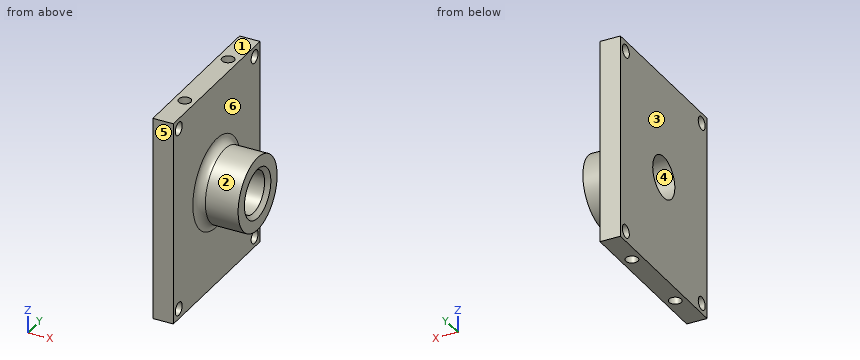
Autodesk Inventor part; units mm, degrees
ref_plane "YZ Plane" through (0, 0, 0) normal (1, 0, 0) x (0, 1, 0)
ref_plane "XZ Plane" through (0, 0, 0) normal (0, 1, 0) x (-1, 0, 0)
ref_plane "XY Plane" through (0, 0, 0) normal (0, 0, 1) x (1, 0, 0)
sketch "Sketch1" plane through (0, 0, 0) normal (1, 0, 0) x (0, 1, 0)
  line L0 (20, 25) -> (-20, 25)
  line L1 (-20, 25) -> (-20, -25)
  line L2 (-20, -25) -> (20, -25)
  line L3 (20, -25) -> (20, 25)
  point P0 (0, 0)
  dimension "d0" = 40
  dimension "d1" = 50
  dimension "d2" = 20
  dimension "d3" = 25
extrude "Extrusion1" add sketch "Sketch1" along normal blind 5
sketch "Sketch2" plane through (5, 0, 0) normal (1, 0, 0) x (0, 0, -1)
  circle A0 centre (0, 0) radius 5.1
  dimension "d6" = 10.2
extrude "Extrusion2" cut sketch "Sketch2" against normal through all
sketch "Sketch3" plane through (5, 0, 0) normal (1, 0, 0) x (0, 0, -1)
  circle A0 centre (0, 0) radius 5.1
  circle A1 centre (0, 0) radius 9
  dimension "d9" = 10.2
  dimension "d10" = 18
extrude "Extrusion3" add sketch "Sketch3" along normal blind 10
chamfer "Chamfer1" distance 1 angle 45 1 edges at (15, 0, 5.1)
fillet "Fillet1" radius 2 1 edges at (5, 0, 9)
sketch "Sketch4" plane through (5, 0, 0) normal (1, 0, 0) x (0, 0, -1)
  circle A0 centre (-22.5, 17.5) radius 1.6
  circle A1 centre (22.5, 17.5) radius 1.6
  circle A2 centre (22.5, -17.5) radius 1.6
  circle A3 centre (-22.5, -17.5) radius 1.6
  line L0 (-25, 20) -> (-25, -20)
  line L1 (25, 20) -> (-25, 20)
  line L2 (25, -20) -> (25, 20)
  line L3 (-25, -20) -> (25, -20)
  point P0 (0, 0)
  dimension "d17" = 3.2
  dimension "d18" = 3.2
  dimension "d19" = 3.2
  dimension "d20" = 3.2
  dimension "d21" = 2.5
  dimension "d22" = 2.5
  dimension "d23" = 2.5
  dimension "d24" = 2.5
  dimension "d25" = 2.5
  dimension "d26" = 2.5
  dimension "d27" = 2.5
  dimension "d28" = 2.5
extrude "Extrusion4" cut sketch "Sketch4" against normal through all contours A0 | A1 | A2 | A3
sketch "Sketch5" plane through (0, -20, 25) normal (0, 0, 1) x (1, 0, 0)
  circle A0 centre (2.5, 30) radius 1.5
  line L0 (0, 40) -> (0, 0)
  circle A1 centre (2.5, 10) radius 1.5
  point P0 (0, 20)
  point P1 (0, 20)
  point P2 (0, 20)
  dimension "d31" = 3
  dimension "d32" = 2.5
  dimension "d33" = 10
  dimension "d34" = 3
  dimension "d35" = 2.5
  dimension "d36" = 10
extrude "Extrusion5" cut sketch "Sketch5" against normal blind 5
mirror "Mirror1" about plane through (0, 0, 0) normal (0, 0, 1) of "Extrusion5"
properties part number "Handle_Front_End" material "ABS Plastic"
Verification items for the finished model (mm, model axes). Face numbers are marked on the shaded views. A direction names the side the tool comes from. Coordinates: 2 decimals unless noted, no trailing zeros. Write each loop counter-clockwise with the first axis right and the second up, starting at its lowest first coordinate (ties: lowest second). Pieces come first, ordered by that corner, then holes. Notation, with made-up numbers: (26.5, 38) - (47.5, 38) arc R23 ccw to (47.5, 73) - close; hole circle Ø2 at (-33.75, -23). An arc over 180 degrees is marked (long way). One line per question, with ' | ' between items. Start each with the question number.
1. Draft check along Z on the marked faces 1, 2, 3 and 4. Enter one of: released by +Z, released by -Z, zero draft, split by the parting line, or undercut.
2. Material ranges on line 1 along Y through (x, z) = (2.5, -22.45); line 2 along Y through (x, z) = (2.5, -21.85); line 3 along X through (y, z) = (-15, -13.5), recorded low to high.
3. Section check D-D (x = 2.5). Enter the section's corners in (y, z), plus the area to 3 significant figures.
4. Section check B-B (y = 0). Enter the section's corners in (x, z), plus the area to 3 significant figures.
5. Gauge pin test, flat ends, axial feed: P1, Ø12, axis at y = 13, z = 9, coming from the +X side; P2, Ø0.9, axis at x = 2.5, y = -10, coming from the +Z side; P3, Ø5, axis at y = -17.5, z = 22.5, coming from the +X side. Record the tip position at first contact, or that the pin passes through.
6. Access from +Z, -Z, +X, -X, +Y, -Y to the whole of each face (thin tool, end or side, straight path). Record for the marked faces 5 and 6.
7. Section check A-A (z = -22.5). Enter the section's corners in (x, y), plus the area to 3 significant figures.
8. Section check C-C (z = 0). Enter the section's corners in (x, y), plus the area to 3 significant figures.
Computed values:
1) face 1: released by +Z | face 2: split by the parting line | face 3: zero draft | face 4: undercut
2) line 1: -20 to -19.1, -15.9 to -11.5, -8.5 to 8.5, 11.5 to 15.9, 19.1 to 20 | line 2: -20 to -18.96, -16.04 to -11.5, -8.5 to 8.5, 11.5 to 16.04, 18.96 to 20 | line 3: 0 to 5
3) outline: (-20, -25) - (-11.5, -25) - (-11.5, -20) - (-8.5, -20) - (-8.5, -25) - (8.5, -25) - (8.5, -20) - (11.5, -20) - (11.5, -25) - (20, -25) - (20, 25) - (11.5, 25) - (11.5, 20) - (8.5, 20) - (8.5, 25) - (-8.5, 25) - (-8.5, 20) - (-11.5, 20) - (-11.5, 25) - (-20, 25) - close; hole circle Ø3.2 at (-17.5, -22.5); hole circle Ø3.2 at (-17.5, 22.5); hole circle Ø10.2 at (0, 0); hole circle Ø3.2 at (17.5, -22.5); hole circle Ø3.2 at (17.5, 22.5) | area: 1,830 mm²
4) outline: (0, -25) - (5, -25) - (5, -11) arc R2 cw to (7, -9) - (15, -9) - (15, -6.1) - (14, -5.1) - (0, -5.1) - close; (0, 5.1) - (14, 5.1) - (15, 6.1) - (15, 9) - (7, 9) arc R2 cw to (5, 11) - (5, 25) - (0, 25) - close | area: 278 mm²
5) P1: x = 5.39 | P2: z = 20 | P3: x = 5
6) face 5: +Z, -Z, +X, -X, -Y | face 6: +X
7) outline: (0, -20) - (5, -20) - (5, -19.1) - (0, -19.1) - close; (0, -15.9) - (5, -15.9) - (5, 15.9) - (0, 15.9) - close; (0, 19.1) - (5, 19.1) - (5, 20) - (0, 20) - close; hole circle Ø3 at (2.5, -10); hole circle Ø3 at (2.5, 10) | area: 154 mm²
8) outline: (0, -20) - (5, -20) - (5, -11) arc R2 cw to (7, -9) - (15, -9) - (15, -6.1) - (14, -5.1) - (0, -5.1) - close; (0, 5.1) - (14, 5.1) - (15, 6.1) - (15, 9) - (7, 9) arc R2 cw to (5, 11) - (5, 20) - (0, 20) - close | area: 228 mm²
